Autodesk Fusion 360 part; units mm, degrees
sketch "Sketch1" plane through (0, 0, 0) normal (0, 1, 0) x (1, 0, 0)
  line L0 (40, -40) -> (80, -40)
  line L1 (80, -40) -> (80, -80)
  line L2 (80, -80) -> (40, -80)
  line L3 (40, -80) -> (40, -40)
  line L4 (80, -40) -> (100, -40)
  line L5 (100, -40) -> (100, -80)
  line L6 (100, -80) -> (80, -80)
  line L7 (40, -80) -> (20, -80)
  line L8 (20, -80) -> (20, -40)
  line L9 (20, -40) -> (40, -40)
  line L10 (20, -60) -> (100, -60)
  circle A0 centre (20, -60) radius 20
  circle A1 centre (100, -60) radius 20
  circle A2 centre (100, -60) radius 10
  circle A3 centre (20, -60) radius 10
  dimension "d1" = 40
  dimension "d2" = 40
  dimension "d3" = 20
  dimension "d4" = 40
  dimension "d5" = 40
  dimension "d6" = 20
  dimension "d7" = 20
extrude "Extrude1" add sketch "Sketch1" against normal blind 10 contours L0 L1 L3 L10 | L3 L9 A0 | L1 L4 A1 | L1 L2 L3 L10 | L8 L10 A0 A3 | L8 L10 A0 A3 | L3 L7 A0 | L8 A0 A3 | L1 L6 A1 | L5 L10 A1 A2 | L5 L10 A1 A2 | L5 A1 A2
extrude "Extrude2" add sketch "Sketch1" along normal blind 40 contours L0 L1 L3 L10 | L1 L2 L3 L10
fillet "Fillet1" radius 20 1 edges at (80, 40, 60)
fillet "Fillet2" radius 20 1 edges at (40, 40, 60)
sketch "Sketch2" plane through (0, 0, 40) normal (0, 0, -1) x (-1, 0, 0)
  arc A0 (-40, 20) -> (-80, 20) centre (-60, 20) ccw
  line L0 (-80, 20) -> (-80, 0)
  line L1 (-80, 0) -> (-100, 0)
  line L2 (-100, 0) -> (-100, -10)
  line L3 (-100, -10) -> (-20, -10)
  line L4 (-20, -10) -> (-20, 0)
  line L5 (-20, 0) -> (-40, 0)
  line L6 (-40, 0) -> (-40, 20)
  line L7 (-80, 0) -> (-40, 0)
  line L8 (-40, 0) -> (-40, 40)
  line L9 (-40, 40) -> (-80, 40)
  line L10 (-80, 40) -> (-80, 0)
  line L11 (-80, 40) -> (-40, 0)
  line L12 (-80, 0) -> (-40, 40)
  circle A1 centre (-60, 20) radius 10
  dimension "d16" = 40
  dimension "d17" = 40
  dimension "d18" = 20
extrude "Extrude3" cut sketch "Sketch2" against normal blind 40 contours L11 L12 A1 | L11 L12 A1 | L11 L12 A1 | L11 L12 A1
Source: CAD feature listing. Evaluate the final solid. Frame: model axes, mm. A direction names the side the tool comes from. Round coordinates to 2 decimals unless told otherwise and drop trailing zeros. Order: outer loops, then holes, each group sorted by start corner. A loop starts at its lowest first (then second) coordinate and runs counter-clockwise, first axis right, second up. Notation, with made-up numbers: (-6.75, 46) -> (19.25, 46) arc R18 cw to (19.25, 65) -> close; hole circle Ø3 at (42, 0.25). An arc over 180 degrees is marked (long way). Use CSV: the item, a comma, the result in double quotes.
(1) Section A-A on z = 57. Count the separate pieces of the cut face and the enclosed holes in it, and give its area (3 significant figures).
Report:
separate pieces,"3"
enclosed holes,"1"
area,"1,930 mm^2"
(2) First-contact query: pin 1 Ø22 at (y, z) = (13, 54) entering from -X; pin 2 Ø1.5 at (y, z) = (33.5, 49.5) entering from +X; pin 3 Ø12 at (x, z) = (23, 50.5) entering from +Y. Flat tips, straight axial feed; report the tip coordinate or a pass-through.
Report:
pin 1,"x = 40"
pin 2,"x = 75.41"
pin 3,"y = 0"
(3) Pull-direction query (X, two-part tool) for faces 1 (the face through (92, -5, 66)), 2 (the face through (80, 10, 60)), 3 (the face through (40, 10, 60)); classes: +X half, -X half, draft (parallel to the pull), parting line (faces both ways), or undercut.
Report:
face 1,"undercut"
face 2,"+X half"
face 3,"-X half"
(4) Section B-B on x = 25.5. Return the cut outline in (y, z).
Report:
outline,"(-10, 40) -> (0, 40) -> (0, 51.65) -> (-10, 51.65) -> close; (-10, 68.35) -> (0, 68.35) -> (0, 80) -> (-10, 80) -> close"
(5) Ray query, L1, parallel to X at y = -3.5, z = 60; L2, parallel to X at y = 20, z = 64.5; L3, parallel to Y at x = 60, z = 56. Return the intervals inside material, ascending.
Report:
L1,"0 to 10, 30 to 90, 110 to 120"
L2,"40 to 50, 70 to 80"
L3,"-10 to 10, 30 to 40"
(6) Section C-C on y = 16.5. Return the cut outline in (x, z).
Report:
outline,"(40, 40) -> (50.63, 40) -> (50.63, 80) -> (40, 80) -> close; (69.37, 40) -> (80, 40) -> (80, 80) -> (69.37, 80) -> close"
(7) Access query for faces 4 (the face through (33, 0, 60)), 5 (the face through (59, -10, 60)), 6 (the face through (91, 0, 55)). Directions: +Z, -Z, +X, -X, +Y, -Y. A direction counts if a zero-diameter tool reaches every point of the face in a straight line with its end or side. Return the directions, or none.
Report:
face 4,"+Z, -Z, -X, +Y"
face 5,"+Z, -Z, +X, -X, -Y"
face 6,"+Z, -Z, +X, +Y"
